Check sheet for the modelled part. Datum: model origin and axes. Units: mm. Face numbers are marked on the shaded views. A direction names the side the tool comes from. Give positions to 0.01 mm unless a question says otherwise; leave off trailing zeros. Order: outer loops, then holes, each group sorted by start corner. A loop starts at its lowest first (then second) coordinate and runs counter-clockwise, first axis right, second up.
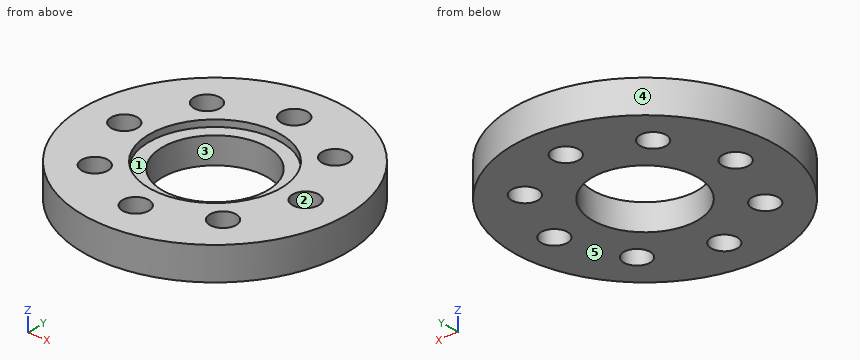
Autodesk Inventor part; units mm, degrees
ref_plane "YZ Plane" through (0, 0, 0) normal (1, 0, 0) x (0, 1, 0)
ref_plane "XZ Plane" through (0, 0, 0) normal (0, 1, 0) x (-1, 0, 0)
ref_plane "XY Plane" through (0, 0, 0) normal (0, 0, 1) x (1, 0, 0)
sketch "スケッチ1" plane through (0, 0, 0) normal (0, 0, 1) x (1, 0, 0)
  circle A0 centre (0, 0) radius 10
  dimension "d0" = 20
extrude "押し出し1" add sketch "スケッチ1" along normal blind 2.5
sketch "スケッチ2" plane through (0, 0, 2.5) normal (0, 0, 1) x (1, 0, 0)
  circle A0 centre (0, 0) radius 10
  circle A1 centre (0, 0) radius 5
  dimension "d3" = 10
hole "穴2" at (0, 0, 2.5) direction (0, 0, -1) diameter 10 depth 0.5
sketch "スケッチ4" plane through (0, 0, 2) normal (0, 0, 1) x (1, 0, 0)
  circle A0 centre (0, 0) radius 5
  circle A1 centre (0, 0) radius 4
  dimension "d21" = 8
hole "穴3" at (0, 0, 2) direction (0, 0, -1) diameter 8 end through all
sketch "スケッチ5" plane through (0, 0, 2.5) normal (0, 0, 1) x (1, 0, 0)
  circle A0 centre (0, 0) radius 5
  circle A1 centre (0, 7) radius 1
  dimension "d29" = 7
  dimension "d30" = 2
hole "穴4" at (0, 7, 2.5) direction (0, 0, -1) diameter 2 end through all
pattern_circular "円形状パターン1" count 8 over 360 about axis through (0, 0, 2.25) along (0, 0, 1) of "穴4"
thread "ねじ1"
thread "ねじ2"
thread "ねじ3"
thread "ねじ4"
thread "ねじ5"
thread "ねじ6"
thread "ねじ7"
thread "ねじ8"
properties part number "03" material "アルミニウム 6061"
(1) Sectioned sample at A-A (y = 0). Enter the section's corners in (x, z).
(2) Go/stop test with flat-tipped pins: P1, Ø1, axis at y = -6, z = 1.5, coming from the -X side; P2, Ø5, axis at x = 1.5, y = 1.5, coming from the +Z side. Record where each tip stops, or that it passes through.
(3) Tool access check on the marked faces 1 and 2. Record the directions out of +Z, -Z, +X, -X, +Y, -Y that give a thin tool (end or side, any length) a straight path to the whole face; none if there is none.
(4) Release check for a two-part mould opening along Y. For the marked faces 3, 4 and 5 record: released by +Y, released by -Y, zero draft, split by the parting line, or undercut.
(5) Thickness scan on L1, parallel to Y at x = 5.5, z = 0.95; L2, parallel to Y at x = 0.25, z = 1.4; L3, parallel to X at y = -4.5, z = 1.9. Record the ranges inside material, lowest first.
(6) Sectioned sample at C-C (z = 0.9). Count the separate pieces of the cut face and the enclosed holes in it, plus the area to 3 significant figures.
(7) Sectioned sample at D-D (x = 7). Enter the section's corners in (y, z), plus the area to 3 significant figures.
Values follow:
1. outline: (-10, 0) - (-8, 0) - (-8, 2.5) - (-10, 2.5) - close; (-6, 0) - (-4, 0) - (-4, 2) - (-5, 2) - (-5, 2.5) - (-6, 2.5) - close; (4, 0) - (6, 0) - (6, 2.5) - (5, 2.5) - (5, 2) - (4, 2) - close; (8, 0) - (10, 0) - (10, 2.5) - (8, 2.5) - close
2. P1: stops at x = -8.35
2. P2: stops at z = 2
3. face 1: +Z
3. face 2: +Z, -Z
4. face 3: undercut
4. face 4: split by the parting line
4. face 5: zero draft
5. L1: y = -8.35 to -5.78, -4.11 to 4.11, 5.78 to 8.35
5. L2: y = -10 to -7.97, -6.03 to -3.99, 3.99 to 6.03, 7.97 to 10
5. L3: x = -8.93 to -5.84, -4.06 to 4.06, 5.84 to 8.93
6. separate pieces: 1
6. enclosed holes: 9
6. area: 239 mm2
7. outline: (-7.14, 0) - (-1, 0) - (-1, 2.5) - (-7.14, 2.5) - close; (1, 0) - (7.14, 0) - (7.14, 2.5) - (1, 2.5) - close
7. area: 30.7 mm2
